from build123d import *

# Parameters (mm, degrees)
F1_DEPTH = 20
F2_SIZE  = 19.99999


# Not quite as in the source:
# - a fillet or chamfer is up to 0.001 mm smaller than in the source, because OpenCascade refuses the exact size


with BuildPart() as f1:
    # F0 (on Top) → F1 (new body)
    with BuildSketch(Plane.XY):
        Polygon((54.2228519917, 569.4585297257), (-1245.7771480083, 569.4585297257), (-1245.7771480083, 14.4585297257), (-1200.7771480083, 14.4585297257), (-1200.7771480083, -30.5414702743), (9.2228519917, -30.5414702743), (9.2228519917, 14.4585297257), (54.2228519917, 14.4585297257), align=None)
    extrude(amount=-F1_DEPTH)

    # F2 (size 20 in the source; OpenCascade refuses exactly that, so slightly less here)
    f2_edges = [f1.edges().sort_by_distance(p)[0] for p in [
        (-1245.777148, 291.95853, -20),
        (54.222852, 291.95853, -20),
    ]]
    chamfer(f2_edges, length=F2_SIZE)


solid = f1.part
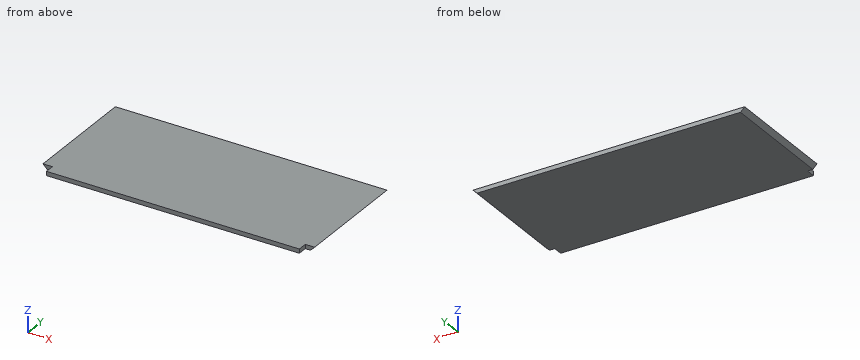
Work out the finished part from the listing and answer in its coordinate system (mm). Give positions to 0.01 mm unless a question says otherwise; leave off trailing zeros. Write each loop counter-clockwise with the first axis right and the second up, starting at its lowest first coordinate (ties: lowest second). Pieces come first, ordered by that corner, then holes.
Q1. Straight lines are drawn through the part: L1, parallel to X at y = 459, z = -12.5; L2, parallel to X at y = 445, z = -19. For each, find the intervals that lie inside material, in ascending order.
Answer:
L1: x = -1233.28 to 41.72
L2: x = -1226.78 to 35.22
Q2. Given pin 1 (12 mm diameter, centred on y = 399.5, z = -17.5, fed in from +X); pin 2 (8 mm diameter, centred on y = 407.5, z = -7, fed in from -X); pin 3 (4 mm diameter, centred on y = 77.5, z = -7.5, fed in from +X), each flat-ended and moving along its own axis, determine where each tip first touches the part or whether it passes through.
Answer:
pin 1: stops at x = 42.72
pin 2: stops at x = -1242.78
pin 3: stops at x = 48.72
Q3. The part is cut by section A-A on z = -15.5. Give the vertices of the cut face in (x, y).
Answer:
outline: (-1230.28, 14.46) - (-1200.78, 14.46) - (-1200.78, -30.54) - (9.22, -30.54) - (9.22, 14.46) - (38.72, 14.46) - (38.72, 569.46) - (-1230.28, 569.46) - close
